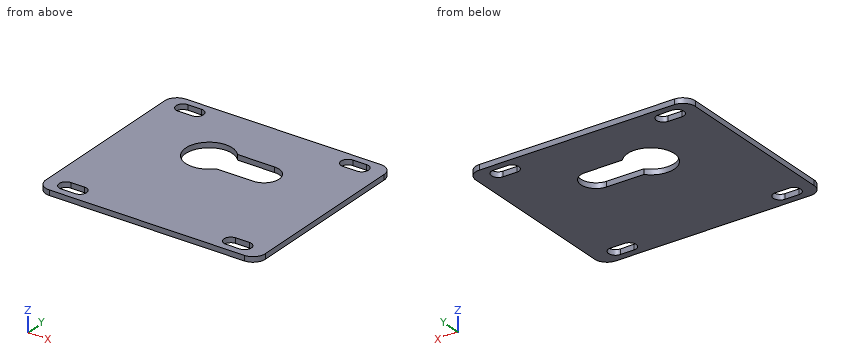
```python
from build123d import *

# Parameters (mm, degrees)
BASE_FLANGE1_START = -1.9
BASE_FLANGE1_DEPTH = 1.9
CUT_EXTRUDE1_DEPTH = 10


# Read off the part's stored shape, not the designer's step: Base-Flange1
with BuildPart() as part:
    # Base-Flange1 outline → Base-Flange1 (new body)
    with BuildSketch(Plane.XY.offset(BASE_FLANGE1_START)):
        with BuildLine():
            Line((39.242670298, -40.5), (39.242670298, 20.5))
            ThreePointArc((39.242670298, 20.5), (37.924650813, 23.681980515), (34.742670298, 25))
            Line((34.742670298, 25), (-36.257329702, 25))
            ThreePointArc((-36.257329702, 25), (-39.439310218, 23.681980516), (-40.757329702, 20.5))
            Line((-40.757329702, 20.5), (-40.757329702, -40.5))
            ThreePointArc((-40.757329702, -40.5), (-39.439310218, -43.681980516), (-36.257329702, -45))
            Line((-36.257329702, -45), (34.742670298, -45))
            ThreePointArc((34.742670298, -45), (37.924650813, -43.681980515), (39.242670298, -40.5))
        make_face()
        with BuildLine():
            ThreePointArc((-33.7157381, -42.5), (-36.2157381, -40), (-33.7157381, -37.5))
            Line((-33.7157381, -37.5), (-28.7157381, -37.5))
            ThreePointArc((-28.7157381, -37.5), (-26.2157381, -40), (-28.7157381, -42.5))
            Line((-28.7157381, -42.5), (-33.7157381, -42.5))
        make_face(mode=Mode.SUBTRACT)
        with BuildLine():
            ThreePointArc((26.2942619, -42.5), (23.7942619, -40), (26.2942619, -37.5))
            Line((26.2942619, -37.5), (31.2942619, -37.5))
            ThreePointArc((31.2942619, -37.5), (33.7942619, -40), (31.2942619, -42.5))
            Line((31.2942619, -42.5), (26.2942619, -42.5))
        make_face(mode=Mode.SUBTRACT)
        with BuildLine():
            ThreePointArc((-33.7157381, 17.5), (-36.2157381, 20), (-33.7157381, 22.5))
            Line((-33.7157381, 22.5), (-28.7157381, 22.5))
            ThreePointArc((-28.7157381, 22.5), (-26.2157381, 20), (-28.7157381, 17.5))
            Line((-28.7157381, 17.5), (-33.7157381, 17.5))
        make_face(mode=Mode.SUBTRACT)
        with BuildLine():
            ThreePointArc((26.394136238, 17.5), (23.894136238, 20), (26.394136238, 22.5))
            Line((26.394136238, 22.5), (31.394136238, 22.5))
            ThreePointArc((31.394136238, 22.5), (33.894136238, 20), (31.394136238, 17.5))
            Line((31.394136238, 17.5), (26.394136238, 17.5))
        make_face(mode=Mode.SUBTRACT)
    extrude(amount=BASE_FLANGE1_DEPTH)

    # Sketch6 → Cut-Extrude1 (cut)
    with BuildSketch(Plane.XY):
        with BuildLine():
            Line((10, 5.5), (-3.519259302, 5.5))
            ThreePointArc((-3.519259302, 5.5), (-18.5, 0), (-3.519259302, -5.5))
            Line((-3.519259302, -5.5), (10, -5.5))
            ThreePointArc((10, -5.5), (15.5, 0), (10, 5.5))
        make_face()
    extrude(amount=-CUT_EXTRUDE1_DEPTH, mode=Mode.SUBTRACT)


solid = part.part
```
The model under review builds one solid part; all positions refer to its coordinate system, in mm. Round coordinates to 2 decimals unless told otherwise and drop trailing zeros. Order: outer loops, then holes, each group sorted by start corner. A loop starts at its lowest first (then second) coordinate and runs counter-clockwise, first axis right, second up. Notation, with made-up numbers: (11, -27.5) -> (45, -27.5) arc R11 ccw to (45, -11.5) -> close; hole circle Ø10 at (-29, -5). An arc over 180 degrees is marked (long way). One line per item, written item: value. Start each with the question number.
Q1. Take a section at A-A (x = -10). Write out the cut boundary in (y, z).
Q2. Take a section at C-C (z = -1.2). Write out the cut boundary in (x, y).
Q3. Wall thickness on line 1 (Y direction, x = 29, z = -0.25); line 2 (Y direction, x = 1.5, z = -1.65); line 3 (Y direction, x = -10, z = -0.35): over which ranges is each line inside the solid? List them lowest first.
Q4. Take a section at B-B (y = 0). Write out the cut boundary in (x, z).
Reported:
1. outline: (-45, -1.9) -> (-8.5, -1.9) -> (-8.5, 0) -> (-45, 0) -> close; (8.5, -1.9) -> (25, -1.9) -> (25, 0) -> (8.5, 0) -> close
2. outline: (-40.76, -40.5) arc R4.5 ccw to (-36.26, -45) -> (34.74, -45) arc R4.5 ccw to (39.24, -40.5) -> (39.24, 20.5) arc R4.5 ccw to (34.74, 25) -> (-36.26, 25) arc R4.5 ccw to (-40.76, 20.5) -> close; hole (-33.72, -42.5) -> (-28.72, -42.5) arc R2.5 ccw to (-28.72, -37.5) -> (-33.72, -37.5) arc R2.5 ccw to start; hole (-33.72, 17.5) -> (-28.72, 17.5) arc R2.5 ccw to (-28.72, 22.5) -> (-33.72, 22.5) arc R2.5 ccw to start; hole (-3.52, -5.5) -> (10, -5.5) arc R5.5 ccw to (10, 5.5) -> (-3.52, 5.5) arc R8.5 ccw (long way) to start; hole (26.29, -42.5) -> (31.29, -42.5) arc R2.5 ccw to (31.29, -37.5) -> (26.29, -37.5) arc R2.5 ccw to start; hole (26.39, 17.5) -> (31.39, 17.5) arc R2.5 ccw to (31.39, 22.5) -> (26.39, 22.5) arc R2.5 ccw to start
3. line 1: y = -45 to -42.5, -37.5 to 17.5, 22.5 to 25
3. line 2: y = -45 to -5.5, 5.5 to 25
3. line 3: y = -45 to -8.5, 8.5 to 25
4. outline: (-40.76, -1.9) -> (-18.5, -1.9) -> (-18.5, 0) -> (-40.76, 0) -> close; (15.5, -1.9) -> (39.24, -1.9) -> (39.24, 0) -> (15.5, 0) -> close
